Read the model definition and answer for the solid it produces. Units are mm, in the model's axes. A direction names the side the tool comes from. Coordinates: 2 decimals unless noted, no trailing zeros. Write each loop counter-clockwise with the first axis right and the second up, starting at its lowest first coordinate (ties: lowest second). Pieces come first, ordered by that corner, then holes.
(1) Section A-A on x = 13.25 is taken. Write down the section's boundary in (y, z).
(2) Given pin 1 (5 mm diameter, centred on x = 18.5, y = -4, fed in from -Z); pin 2 (5 mm diameter, centred on y = -1.5, z = -4.5, fed in from +X); pin 3 (2 mm diameter, centred on y = -2, z = 3, fed in from +X); pin 4 (1 mm diameter, centred on y = -4, z = -3, fed in from -X), each flat-ended and moving along its own axis, determine where each tip first touches the part or whether it passes through.
(3) Which of the six approach directions +Z, -Z, +X, -X, +Y, -Y give full straight-line access (tool end or side, diameter ignored) to faces 1 (the flat face through (14, -5, -4)), 2 (the flat face through (12.586, -4.93, 2.806)), 3 (the flat face through (12.57, -4.93, -2.82)), 4 (the flat face through (19.507, -4.93, -2.713)), 5 (the flat face through (20.31, -4.93, 1.05))?
(4) Find the intervals of material crossed by probe 1 along Z at (x, y) = (19.5, -0.75); probe 2 along Z at (x, y) = (19, -9); probe 3 along X at (y, z) = (-6.75, 4.25), in increasing order.
(5) The mould has two halves that part along X. Classify faces 6 (the flat face through (17.86, -4.93, -4.01)), 7 (the flat face through (16, 0, 0)), 8 (the flat face through (19.495, -4.93, 2.704)), 9 (the flat face through (17.865, -4.93, 4.023)): +X half, -X half, draft (parallel to the pull), parting line (faces both ways), or undercut.
from build123d import *

# Parameters (mm, degrees)
PAD003_DEPTH = 10
POCKET_DEPTH = 10.001


with BuildPart() as obj1:
    # InvoluteGear001 → Pad003 (new body)
    with BuildSketch(Plane(origin=(16, 0, 0), x_dir=(1, 0, 0), z_dir=(0, -1, 0))):
        with BuildLine():
            Line((3.786059, -0.923719), (4.81556, -1.173313))
            add(Edge.make_bspline(
                [(4.81556, -1.173313), (4.873385, -1.181675), (5.046346, -1.195856), (5.34323, -1.127243)],
                knots=[0, 0, 0, 0, 1, 1, 1, 1], degree=3))
            add(Edge.make_bspline(
                [(5.34323, -1.127243), (5.693315, -1.042189), (6.183331, -0.841463), (6.742255, -0.380782)],
                knots=[0, 0, 0, 0, 1, 1, 1, 1], degree=3))
            ThreePointArc((6.742255, -0.380782), (6.753004, 0), (6.742255, 0.380782))
            add(Edge.make_bspline(
                [(6.742255, 0.380782), (6.183331, 0.841463), (5.693315, 1.042189), (5.34323, 1.127243)],
                knots=[0, 0, 0, 0, 1, 1, 1, 1], degree=3))
            add(Edge.make_bspline(
                [(5.34323, 1.127243), (5.046346, 1.195856), (4.873385, 1.181675), (4.81556, 1.173313)],
                knots=[0, 0, 0, 0, 1, 1, 1, 1], degree=3))
            Line((4.81556, 1.173313), (3.786059, 0.923719))
            ThreePointArc((3.786059, 0.923719), (3.397937, 0.968687), (3.132738, 1.25562))
            ThreePointArc((3.132738, 1.25562), (3.04077, 1.464358), (2.934913, 1.666407))
            ThreePointArc((2.934913, 1.666407), (2.875929, 2.052647), (3.082762, 2.384131))
            Line((3.082762, 2.384131), (3.919786, 3.033407))
            add(Edge.make_bspline(
                [(3.919786, 3.033407), (3.962376, 3.073404), (4.081304, 3.199788), (4.212764, 3.474681)],
                knots=[0, 0, 0, 0, 1, 1, 1, 1], degree=3))
            add(Edge.make_bspline(
                [(4.212764, 3.474681), (4.364539, 3.801419), (4.513126, 4.309679), (4.501435, 5.033894)],
                knots=[0, 0, 0, 0, 1, 1, 1, 1], degree=3))
            ThreePointArc((4.501435, 5.033894), (4.210429, 5.279711), (3.90602, 5.508721))
            add(Edge.make_bspline(
                [(3.90602, 5.508721), (3.197362, 5.358966), (2.734908, 5.101007), (2.450135, 4.88033)],
                knots=[0, 0, 0, 0, 1, 1, 1, 1], degree=3))
            add(Edge.make_bspline(
                [(2.450135, 4.88033), (2.211387, 4.690996), (2.114635, 4.546928), (2.085119, 4.496505)],
                knots=[0, 0, 0, 0, 1, 1, 1, 1], degree=3))
            Line((2.085119, 4.496505), (1.638377, 3.53599))
            ThreePointArc((1.638377, 3.53599), (1.361229, 3.260581), (0.971547, 3.232139))
            ThreePointArc((0.971547, 3.232139), (0.751008, 3.290382), (0.527039, 3.333595))
            ThreePointArc((0.527039, 3.333595), (0.188288, 3.528297), (0.058082, 3.896681))
            Line((0.058082, 3.896681), (0.072333, 4.95591))
            add(Edge.make_bspline(
                [(0.072333, 4.95591), (0.067617, 5.014146), (0.042956, 5.185927), (-0.09, 5.460099)],
                knots=[0, 0, 0, 0, 1, 1, 1, 1], degree=3))
            add(Edge.make_bspline(
                [(-0.09, 5.460099), (-0.250823, 5.78248), (-0.555555, 6.215545), (-1.129058, 6.657945)],
                knots=[0, 0, 0, 0, 1, 1, 1, 1], degree=3))
            ThreePointArc((-1.129058, 6.657945), (-1.502685, 6.583692), (-1.871528, 6.488481))
            add(Edge.make_bspline(
                [(-1.871528, 6.488481), (-2.196286, 5.841059), (-2.28294, 5.318663), (-2.287961, 4.958429)],
                knots=[0, 0, 0, 0, 1, 1, 1, 1], degree=3))
            add(Edge.make_bspline(
                [(-2.287961, 4.958429), (-2.288791, 4.65372), (-2.236478, 4.488252), (-2.215459, 4.433737)],
                knots=[0, 0, 0, 0, 1, 1, 1, 1], degree=3))
            Line((-2.215459, 4.433737), (-1.743037, 3.485588))
            ThreePointArc((-1.743037, 3.485588), (-1.700512, 3.09719), (-1.921238, 2.774792))
            ThreePointArc((-1.921238, 2.774792), (-2.104278, 2.638681), (-2.277706, 2.490518))
            ThreePointArc((-2.277706, 2.490518), (-2.641138, 2.347067), (-3.010335, 2.474951))
            Line((-3.010335, 2.474951), (-3.829588, 3.146512))
            add(Edge.make_bspline(
                [(-3.829588, 3.146512), (-3.878059, 3.179135), (-4.027738, 3.266957), (-4.324991, 3.333952)],
                knots=[0, 0, 0, 0, 1, 1, 1, 1], degree=3))
            add(Edge.make_bspline(
                [(-4.324991, 3.333952), (-4.677311, 3.409216), (-5.205892, 3.440979), (-5.909347, 3.268428)],
                knots=[0, 0, 0, 0, 1, 1, 1, 1], degree=3))
            ThreePointArc((-5.909347, 3.268428), (-6.084247, 2.930019), (-6.239777, 2.582282))
            add(Edge.make_bspline(
                [(-6.239777, 2.582282), (-5.936086, 1.924715), (-5.581688, 1.531257), (-5.303176, 1.30273)],
                knots=[0, 0, 0, 0, 1, 1, 1, 1], degree=3))
            add(Edge.make_bspline(
                [(-5.303176, 1.30273), (-5.065463, 1.112098), (-4.903478, 1.04983), (-4.847751, 1.032274)],
                knots=[0, 0, 0, 0, 1, 1, 1, 1], degree=3))
            Line((-4.847751, 1.032274), (-3.811908, 0.810467))
            ThreePointArc((-3.811908, 0.810467), (-3.481733, 0.601552), (-3.367292, 0.22797))
            ThreePointArc((-3.367292, 0.22797), (-3.375, 0), (-3.367292, -0.22797))
            ThreePointArc((-3.367292, -0.22797), (-3.481733, -0.601552), (-3.811908, -0.810467))
            Line((-3.811908, -0.810467), (-4.847751, -1.032274))
            add(Edge.make_bspline(
                [(-4.847751, -1.032274), (-4.903478, -1.04983), (-5.065463, -1.112098), (-5.303176, -1.30273)],
                knots=[0, 0, 0, 0, 1, 1, 1, 1], degree=3))
            add(Edge.make_bspline(
                [(-5.303176, -1.30273), (-5.581688, -1.531257), (-5.936086, -1.924715), (-6.239777, -2.582282)],
                knots=[0, 0, 0, 0, 1, 1, 1, 1], degree=3))
            ThreePointArc((-6.239777, -2.582282), (-6.084247, -2.930019), (-5.909347, -3.268428))
            add(Edge.make_bspline(
                [(-5.909347, -3.268428), (-5.205892, -3.440979), (-4.677311, -3.409216), (-4.324991, -3.333952)],
                knots=[0, 0, 0, 0, 1, 1, 1, 1], degree=3))
            add(Edge.make_bspline(
                [(-4.324991, -3.333952), (-4.027738, -3.266957), (-3.878059, -3.179135), (-3.829588, -3.146512)],
                knots=[0, 0, 0, 0, 1, 1, 1, 1], degree=3))
            Line((-3.829588, -3.146512), (-3.010335, -2.474951))
            ThreePointArc((-3.010335, -2.474951), (-2.641138, -2.347067), (-2.277706, -2.490518))
            ThreePointArc((-2.277706, -2.490518), (-2.104278, -2.638681), (-1.921238, -2.774792))
            ThreePointArc((-1.921238, -2.774792), (-1.700512, -3.09719), (-1.743037, -3.485588))
            Line((-1.743037, -3.485588), (-2.215459, -4.433737))
            add(Edge.make_bspline(
                [(-2.215459, -4.433737), (-2.236478, -4.488252), (-2.288791, -4.65372), (-2.287961, -4.958429)],
                knots=[0, 0, 0, 0, 1, 1, 1, 1], degree=3))
            add(Edge.make_bspline(
                [(-2.287961, -4.958429), (-2.28294, -5.318663), (-2.196286, -5.841059), (-1.871528, -6.488481)],
                knots=[0, 0, 0, 0, 1, 1, 1, 1], degree=3))
            ThreePointArc((-1.871528, -6.488481), (-1.502685, -6.583692), (-1.129058, -6.657945))
            add(Edge.make_bspline(
                [(-1.129058, -6.657945), (-0.555555, -6.215545), (-0.250823, -5.78248), (-0.09, -5.460099)],
                knots=[0, 0, 0, 0, 1, 1, 1, 1], degree=3))
            add(Edge.make_bspline(
                [(-0.09, -5.460099), (0.042956, -5.185927), (0.067617, -5.014146), (0.072333, -4.95591)],
                knots=[0, 0, 0, 0, 1, 1, 1, 1], degree=3))
            Line((0.072333, -4.95591), (0.058082, -3.896681))
            ThreePointArc((0.058082, -3.896681), (0.188288, -3.528297), (0.527039, -3.333595))
            ThreePointArc((0.527039, -3.333595), (0.751008, -3.290382), (0.971547, -3.232139))
            ThreePointArc((0.971547, -3.232139), (1.361229, -3.260581), (1.638377, -3.53599))
            Line((1.638377, -3.53599), (2.085119, -4.496505))
            add(Edge.make_bspline(
                [(2.085119, -4.496505), (2.114635, -4.546928), (2.211387, -4.690996), (2.450135, -4.88033)],
                knots=[0, 0, 0, 0, 1, 1, 1, 1], degree=3))
            add(Edge.make_bspline(
                [(2.450135, -4.88033), (2.734908, -5.101007), (3.197362, -5.358966), (3.90602, -5.508721)],
                knots=[0, 0, 0, 0, 1, 1, 1, 1], degree=3))
            ThreePointArc((3.90602, -5.508721), (4.210429, -5.279711), (4.501435, -5.033894))
            add(Edge.make_bspline(
                [(4.501435, -5.033894), (4.513126, -4.309679), (4.364539, -3.801419), (4.212764, -3.474681)],
                knots=[0, 0, 0, 0, 1, 1, 1, 1], degree=3))
            add(Edge.make_bspline(
                [(4.212764, -3.474681), (4.081304, -3.199788), (3.962376, -3.073404), (3.919786, -3.033407)],
                knots=[0, 0, 0, 0, 1, 1, 1, 1], degree=3))
            Line((3.919786, -3.033407), (3.082762, -2.384131))
            ThreePointArc((3.082762, -2.384131), (2.875929, -2.052647), (2.934913, -1.666407))
            ThreePointArc((2.934913, -1.666407), (3.04077, -1.464358), (3.132738, -1.25562))
            ThreePointArc((3.132738, -1.25562), (3.397937, -0.968687), (3.786059, -0.923719))
        make_face()
    extrude(amount=PAD003_DEPTH)


with BuildPart() as obj1_con_buco:
    # Pocket base: copy of obj1
    add(obj1.part)

    # Sketch012 → Pocket (cut, through all)
    with BuildSketch(Plane(origin=(16, -10, 0), x_dir=(1, 0, 0), z_dir=(0, -1, 0))):
        with BuildLine():
            ThreePointArc((1.075668, -1.045437), (0.009602, 1.50979), (-1.056464, -1.045437))
            Line((-1.056464, -1.045437), (1.075668, -1.045437))
        make_face()
    extrude(amount=-POCKET_DEPTH, mode=Mode.SUBTRACT)

    # Fusion004: union obj1
    add(obj1.part)


solid = obj1_con_buco.part
Response:
1. outline: (-10, -2.36) - (0, -2.36) - (0, 2.36) - (-10, 2.36) - close
2. pin 1: stops at z = -5.51
2. pin 2: stops at x = 20.5
2. pin 3: stops at x = 20.39
2. pin 4: stops at x = 9.76
3. face 1: -X, +Y, -Y
3. face 2: +Z, +Y, -Y
3. face 3: -Z, +Y, -Y
3. face 4: +X, +Y, -Y
3. face 5: +Y, -Y
4. probe 1: z = -5.4 to -2.71, -0.93 to 0.93, 2.71 to 5.4
4. probe 2: z = -5.21 to -2.31, -1.55 to 1.55, 2.31 to 5.21
4. probe 3: x = 13.88 to 16.06, 17.97 to 20.45
5. face 6: undercut
5. face 7: draft
5. face 8: +X half
5. face 9: undercut
